Verification items for this drawing (mm, ordinates from the low corner). A direction names the side the tool comes from. Give positions to 0.01 mm unless a question says otherwise; leave off trailing zeros. Loops run counter-clockwise (first coordinate to the right, second up) from the corner with the lowest first, then second, coordinate; pieces in that order, holes last. Notation, with made-up numbers: (88.25, 42.5) -> (144.25, 42.5) arc R10 cw to (144.25, 56.5) -> close; hole circle Ø3 at (-10.5, -0.5). An arc over 180 degrees is marked (long way). Answer in a Markdown table with one row per item. Add a question column.
Q1. Gauge pin test, flat ends, axial feed: P1, Ø4, axis at y = 129, z = 77, coming from the -X side; P2, Ø8, axis at x = 791, z = 141, coming from the -Y side. Record the tip position at first contact, or that the pin passes through.
Q2. Material ranges on probe 1 along X at (y, z) = (102, 24); probe 2 along Z at (x, y) = (2242, 177.5); probe 3 along Y at (x, z) = (201, 256.5), recorded low to high.
Q3. Section check B-B on z = 235. Enter the section's corners in (x, y), and give its area (3 significant figures).
Q4. Section check C-C on x = 1579. Enter the section's corners in (y, z), and give its area (3 significant figures).
Q5. Section check A-A on y = 126.5. Enter the section's corners in (x, z), and give its area (3 significant figures).
Q6. Release check for a two-part mould opening along Z. For the marked faces 1, 2, 3 and 4 record: pulls with the +Z half, pulls with the -Z half, needs draft (parallel to the pull), parting line crosses it, or undercut.
Q7. Set-up check for the marked faces 5 and 6: record each of +Z, -Z, +X, -X, +Y, -Y from which the full face is reachable in a straight line by a thin tool's end or side.
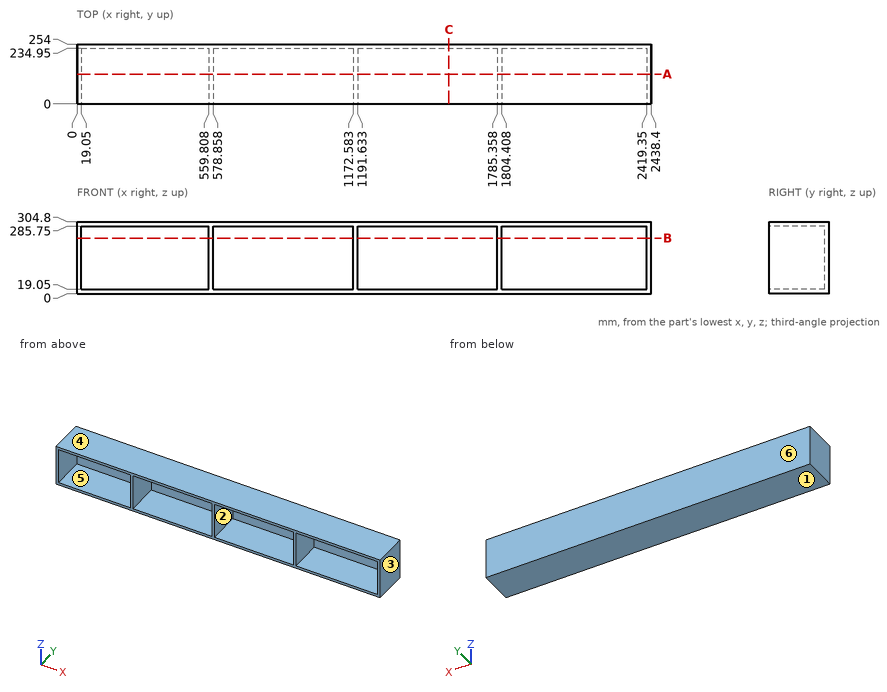
Taken from the geometry:
| question | item | result |
|---|---|---|
| 1 | P1 | stops at x = 0 |
| 1 | P2 | stops at y = 234.95 |
| 2 | probe 1 | x = 0 to 19.05, 559.81 to 578.86, 1172.58 to 1191.63, 1785.36 to 1804.41, 2419.35 to 2438.4 |
| 2 | probe 2 | z = 0 to 19.05, 285.75 to 304.8 |
| 2 | probe 3 | y = 234.95 to 254 |
| 3 | outline | (0, 0) -> (19.05, 0) -> (19.05, 234.95) -> (559.81, 234.95) -> (559.81, 0) -> (578.86, 0) -> (578.86, 234.95) -> (1172.58, 234.95) -> (1172.58, 0) -> (1191.63, 0) -> (1191.63, 234.95) -> (1785.36, 234.95) -> (1785.36, 0) -> (1804.41, 0) -> (1804.41, 234.95) -> (2419.35, 234.95) -> (2419.35, 0) -> (2438.4, 0) -> (2438.4, 254) -> (0, 254) -> close |
| 3 | area | 68,800 mm² |
| 4 | outline | (0, 0) -> (254, 0) -> (254, 304.8) -> (0, 304.8) -> (0, 285.75) -> (234.95, 285.75) -> (234.95, 19.05) -> (0, 19.05) -> close |
| 4 | area | 14,800 mm² |
| 5 | outline | (0, 0) -> (2438.4, 0) -> (2438.4, 304.8) -> (0, 304.8) -> close; hole (19.05, 19.05) -> (559.81, 19.05) -> (559.81, 285.75) -> (19.05, 285.75) -> close; hole (578.86, 19.05) -> (1172.58, 19.05) -> (1172.58, 285.75) -> (578.86, 285.75) -> close; hole (1191.63, 19.05) -> (1785.36, 19.05) -> (1785.36, 285.75) -> (1191.63, 285.75) -> close; hole (1804.41, 19.05) -> (2419.35, 19.05) -> (2419.35, 285.75) -> (1804.41, 285.75) -> close |
| 5 | area | 118,000 mm² |
| 6 | face 1 | pulls with the -Z half |
| 6 | face 2 | undercut |
| 6 | face 3 | needs draft |
| 6 | face 4 | pulls with the +Z half |
| 7 | face 5 | -Y |
| 7 | face 6 | +Z, -Z, +X, -X, +Y |
